Part model, mm, in its own coordinate system. A direction names the side the tool comes from. Give positions to 0.01 mm unless a question says otherwise; leave off trailing zeros. Order: outer loops, then holes, each group sorted by start corner. A loop starts at its lowest first (then second) coordinate and runs counter-clockwise, first axis right, second up. Notation, with made-up numbers: (75.5, -9.75) - (89.5, -9.75) arc R36 ccw to (89.5, 29.25) - close; hole circle Ø9 at (39, 4.25). An arc over 180 degrees is marked (long way). Use a Markdown table: item, result. Add a question column.
Autodesk Inventor part; units mm, degrees
ref_plane "YZ Plane" through (0, 0, 0) normal (1, 0, 0) x (0, 1, 0)
ref_plane "XZ Plane" through (0, 0, 0) normal (0, 1, 0) x (-1, 0, 0)
ref_plane "XY Plane" through (0, 0, 0) normal (0, 0, 1) x (1, 0, 0)
sketch "Sketch1" plane through (0, 0, 0) normal (0, 0, 1) x (1, 0, 0)
  line L0 (-20, 10) -> (20, 10)
  line L1 (20, 10) -> (20, -10)
  line L2 (20, -10) -> (-20, -10)
  line L3 (-20, -10) -> (-20, 10)
  line L4 (-20, 10) -> (20, -10) construction
  line L5 (20, 10) -> (-20, -10) construction
  line L6 (18, 8) -> (-18, 8)
  line L7 (-18, 8) -> (-18, -8)
  line L8 (-18, -8) -> (18, -8)
  line L9 (18, -8) -> (18, 8)
  point P0 (0, 0)
  dimension "d0" = 40
  dimension "d1" = 20
  dimension "d2" = 2
extrude "Extrusion1" add sketch "Sketch1" along normal mid plane 700
sketch "Sketch2" plane through (0, 0, 0) normal (0, 1, 0) x (-1, 0, 0)
  line L0 (20, -350) -> (20, 350)
  line L1 (-20, 350) -> (20, 350)
  line L2 (-20, -350) -> (-20, 350)
  line L3 (20, -350) -> (-20, -350)
  line L4 (-20, -350) -> (-50.7107, -350)
  line L5 (-50.7107, -350) -> (-50.7107, 350)
  line L6 (-50.7107, 350) -> (-20, 350)
  line L7 (20, -279.2893) -> (-50.7107, -350)
  line L8 (20, -279.2893) -> (-20, -262.7208)
  line L9 (-20, -350) -> (-20, 350)
  point P0 (0, 0)
  point P1 (-20, -319.2893)
  dimension "d5" = 45
  dimension "d6" = 100
  dimension "d19" = 67.5
extrude "Extrusion2" cut sketch "Sketch2" along normal through all both and the other way through all contours L3 L2 L7 L0 | L7 L2 L8
mirror "Mirror1" about plane through (0, 0, 0) normal (0, 0, 1) of "Extrusion2"
sketch "Sketch3" plane through (0, 0, 0) normal (0, 1, 0) x (-1, 0, 0)
  line L0 (0, 0) -> (0, -271.0051) construction
  line L1 (-20, -262.7208) -> (-20, 262.7208) construction
  line L2 (20, 279.2893) -> (20, -279.2893) construction
  circle A0 centre (0, -165) radius 5.5
  line L3 (20, 279.2893) -> (20, -279.2893) construction
  line L4 (-20, -262.7208) -> (20, -279.2893) construction
  dimension "d10" = 11
  dimension "d20" = 165
extrude "Extrusion3" cut sketch "Sketch3" along normal through all
mirror "Mirror2" about plane through (0, 0, 0) normal (0, 0, 1) of "Extrusion3"
fillet "Fillet1" radius 2 4 edges at (-20, 10, 0) (-20, -10, 0) (20, -10, 0) (20, 10, 0)
equation "\"d19\" = 1.5 * d5"
properties part number "Long tube 1_CPY"
1. Cut at A-A (y = -1). Write the cut outline in (x, z).
2. Cut at C-C (x = 0). Write the cut outline in (y, z), plus the area to 3 significant figures.
3. Cut at B-B (z = 142.5). Write the cut outline in (x, y), plus the area to 3 significant figures.
4. Mould opens along Y. For faces 4 (the face through (-1.575, -8.195, -271.657)), 5 (the face through (0, 8, -4)), 6 (the face through (0, 10, -4)), 7 (the face through (18, 0, -4)) say: released by +Y, released by -Y, zero draft, split by the parting line, or undercut.
5. Drill centre lines: probe 1 along X at (y, z) = (6.75, -68.5); probe 2 along Y at (x, z) = (7, 251); probe 3 along Z at (x, y) = (0, 8.75). Where is each one in solid material? Low to high. Write a range as [from, to].
6. Pin check, flat tips, straight feed: P1, Ø10, axis at x = 6.5, y = -6.5, coming from the +Z side; P2, Ø10, axis at x = 0, z = -165, coming from the +Y side; P3, Ø17.5, axis at x = 0, z = 165, coming from the +Y side. Stop position of each tip, or through.
7. Tool access for faces 1 (the face through (1.19, 8.99, -159.63)), 2 (the face through (0, -8, -4)), 3 (the face through (0, -10, -4)): list every direction of +Z, -Z, +X, -X, +Y, -Y with a clear straight run to the whole face (end or side of a thin tool).
Responses:
| question | item | result |
|---|---|---|
| 1 | outline | (-20, -279.29) - (-18, -278.46) - (-18, 278.46) - (-20, 279.29) - close; (18, -263.55) - (20, -262.72) - (20, 262.72) - (18, 263.55) - close |
| 2 | outline | (-10, -271.01) - (-8, -271.01) - (-8, 271.01) - (-10, 271.01) - close; (8, -271.01) - (10, -271.01) - (10, -170.5) - (8, -170.5) - close; (8, -159.5) - (10, -159.5) - (10, 159.5) - (8, 159.5) - close; (8, 170.5) - (10, 170.5) - (10, 271.01) - (8, 271.01) - close |
| 2 | area | 2,120 mm² |
| 3 | outline | (-20, -8) arc R2 ccw to (-18, -10) - (18, -10) arc R2 ccw to (20, -8) - (20, 8) arc R2 ccw to (18, 10) - (-18, 10) arc R2 ccw to (-20, 8) - close; hole (-18, -8) - (18, -8) - (18, 8) - (-18, 8) - close |
| 3 | area | 221 mm² |
| 4 | face 4 | zero draft |
| 4 | face 5 | undercut |
| 4 | face 6 | released by +Y |
| 4 | face 7 | undercut |
| 5 | probe 1 | x = [-20, -18], [18, 20] |
| 5 | probe 2 | y = [-10, -8], [8, 10] |
| 5 | probe 3 | z = [-271.01, -170.5], [-159.5, 159.5], [170.5, 271.01] |
| 6 | P1 | stops at z = 270.29 |
| 6 | P2 | stops at y = -8 |
| 6 | P3 | stops at y = 10 |
| 7 | face 1 | +Y |
| 7 | face 2 | +Z, -Z |
| 7 | face 3 | +Z, -Z, +X, -X, -Y |
